Design review of the part built by this model. Coordinates are the model's own, in mm. Give positions to 0.01 mm unless a question says otherwise; leave off trailing zeros. Write each loop counter-clockwise with the first axis right and the second up, starting at its lowest first coordinate (ties: lowest second). Pieces come first, ordered by that corner, then holes. Notation, with made-up numbers: M 87.5,-9.5 L 107.5,-9.5 A34 ccw 107.5,29.5 Z; hole C 44.25,89.25 d2. An arc over 180 degrees is marked long. Use a Markdown table: item, result. Add a question column.
Autodesk Inventor part; units mm, degrees
ref_plane "YZ Plane" through (0, 0, 0) normal (1, 0, 0) x (0, 1, 0)
ref_plane "XZ Plane" through (0, 0, 0) normal (0, 1, 0) x (-1, 0, 0)
ref_plane "XY Plane" through (0, 0, 0) normal (0, 0, 1) x (1, 0, 0)
ref_plane "Work Plane1" through (225, -51.9999, -200.9642) normal (1, 0, 0) x (0, 0, -1)
sketch "Sketch1" plane through (225, -51.9999, -200.9642) normal (1, 0, 0) x (0, 0, -1)
  line L0 (-200.9642, 89.4999) -> (-130.9642, 89.4999)
  line L1 (-130.9642, 89.4999) -> (-130.9642, 14.4999)
  line L2 (-130.9642, 14.4999) -> (-200.9642, 14.4999)
  line L3 (-200.9642, 14.4999) -> (-200.9642, -53.5599)
  line L4 (-200.9642, -53.5599) -> (-122.2497, -53.5599)
  ellipse E0 centre (-122.3295, -48.5209) end of major axis (-118.6887, -52.0634) minor radius 5 (-122.2497, -53.5599) -> (-117.3008, -48.2463) ccw
  line L5 (-117.3008, -48.2463) -> (-117.6163, -43.7662)
  line L6 (-117.6163, -43.7662) -> (-94.1545, -42.114)
  line L7 (-94.1545, -42.114) -> (-81.3155, 140.1971)
  arc A0 (-81.3155, 140.1971) -> (-85.9519, 145.536) centre (-86.3031, 140.5484) ccw
  line L8 (-85.9519, 145.536) -> (-117.6163, 147.7659)
  line L9 (-117.6163, 147.7659) -> (-117.3008, 152.246)
  ellipse E1 centre (-122.3295, 152.5206) end of major axis (-118.6887, 156.0631) minor radius 5 (-117.3008, 152.246) -> (-122.2497, 157.5596) ccw
  line L10 (-122.2497, 157.5596) -> (-200.9642, 157.5596)
  line L11 (-200.9642, 89.4999) -> (-200.9642, 157.5596)
  line L12 (-200.9642, 123.5297) -> (-400.9642, 123.5297)
  line L13 (-400.9642, 123.5297) -> (-400.9642, -76.4703)
  line L14 (-400.9642, -76.4703) -> (-200.9642, -76.4703)
  line L15 (-200.9642, -76.4703) -> (-200.9642, 123.5297)
  line L16 (-348.854, 122.9439) -> (-400.9642, 70.8337)
  line L17 (-347.4398, 123.5297) -> (-273.7448, 123.5297) construction
  arc A1 (-347.4398, 123.5297) -> (-348.854, 122.9439) centre (-347.4398, 121.5297) ccw
  point P0 (-200.9642, 51.9999)
  point P1 (-348.2682, 123.5297)
  dimension "d0" = 200
  dimension "d1" = 200
  dimension "d2" = 135
  dimension "d3" = 2
extrude "Extrusion1" add sketch "Sketch1" against normal blind 100 contours L15 L3 L14 L13 L16 A1 L12 L11 | A1 L16 L13 L12
chamfer "Chamfer1" distance 80 angle 45 1 edges at (175, 71.5299, 200)
properties part number "00_STORMModule"
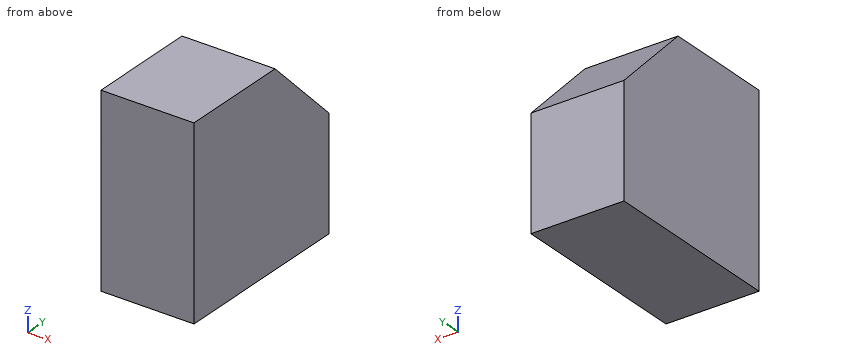
(1) Wall thickness on L1, parallel to Z at x = 168, y = 30; L2, parallel to Y at x = 212, z = 184.5; L3, parallel to Y at x = 161.5, z = 152.5: over which ranges is each line inside the solid? List them lowest first.
(2) For pin 1 (3 mm diameter, centred on x = 210, y = -17.5, fed in from -Z), flat-tipped, find the tip position at first contact; note if it passes through.
(3) Add section A-A on x = 206. Give the boundary of the cut face in (y, z).
From the geometry:
| question | item | result |
|---|---|---|
| 1 | L1 | z = 0 to 161.53 |
| 1 | L2 | y = -128.47 to 7.03 |
| 1 | L3 | y = -128.47 to 39.03 |
| 2 | pin 1 | stops at z = 0 |
| 3 | outline | M -128.47,0 L 71.53,0 L 71.53,120 L -8.47,200 L -128.47,200 Z |
